The listing builds one solid part. Answer for the finished solid, in the listing's coordinates (mm). Face numbers are marked on the shaded views. Coordinates: 2 decimals unless noted, no trailing zeros. Order: outer loops, then holes, each group sorted by start corner. A loop starts at its lowest first (then second) coordinate and runs counter-clockwise, first axis right, second up.
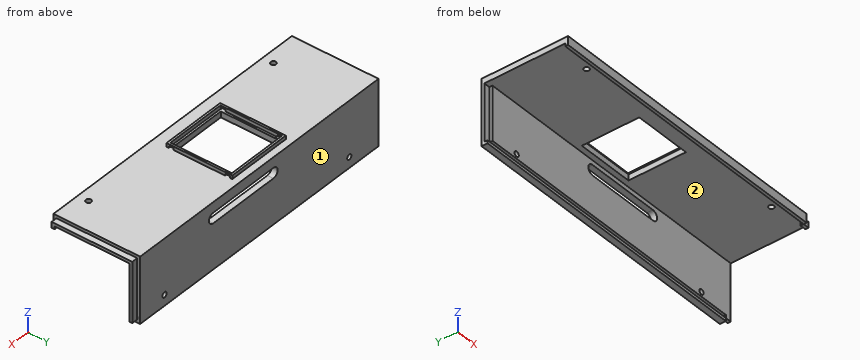
```python
from build123d import *

# Parameters (mm, degrees)
SKETCH_W        = 250
SKETCH_H        = 5
PAD012_DEPTH    = 55
SKETCH023_W     = 2.6
SKETCH023_H     = 2.6
POCKET007_DEPTH = 250.001
SKETCH024_W     = 5.1
SKETCH024_H     = 2.6
POCKET008_DEPTH = 45
SKETCH025_W     = 250
SKETCH025_H     = 4.9
PAD013_DEPTH    = 67.5
SKETCH026_W     = 250
SKETCH026_H     = 2.4
PAD014_DEPTH    = 2.4
SKETCH027_R     = 2.2
HOLE004_DEPTH   = 23.678107
HOLE004_TIPS_R  = 2.2
SKETCH028_R     = 2.2
HOLE005_DEPTH   = 23.678107
HOLE005_TIPS_R  = 2.2
POCKET009_DEPTH = 5
SKETCH030_W     = 48
SKETCH030_H     = 48
POCKET010_DEPTH = 4.9
SKETCH031_W     = 55
SKETCH031_H     = 55
SKETCH031_W_2   = 51.5
SKETCH031_H_2   = 51.5
PAD015_DEPTH    = 3
SKETCH032_W     = 4
SKETCH032_H     = 1.5
POCKET011_DEPTH = 161.951
POCKET012_DEPTH = 5
SKETCH035_W     = 5
SKETCH035_H     = 2.5
PAD016_DEPTH    = 2.6
SKETCH036_W     = 5
SKETCH036_H     = 2.6
PAD017_DEPTH    = 2.4


with BuildPart() as part:
    # Sketch → Pad012 (new body)
    with BuildSketch(Plane.XY):
        with Locations((0, 35)):
            Rectangle(SKETCH_W, SKETCH_H)
    extrude(amount=PAD012_DEPTH)

    # Sketch023 (on Face2 of Pad012) → Pocket007 (cut, through all)
    with BuildSketch(Plane.YZ.offset(125)):
        with Locations((33.8, 3.8)):
            Rectangle(SKETCH023_W, SKETCH023_H)
    extrude(amount=-POCKET007_DEPTH, mode=Mode.SUBTRACT)

    # Sketch024 (on Face7 of Pocket007) → Pocket008 (cut)
    with BuildSketch(Plane(origin=(0, 0, 5.1), x_dir=(1, 0, 0), z_dir=(0, 0, -1))):
        with Locations((-122.45, -33.8)):
            Rectangle(SKETCH024_W, SKETCH024_H)
    extrude(amount=-POCKET008_DEPTH, mode=Mode.SUBTRACT)

    # Sketch025 (on Face6 of Pocket008) → Pad013 (join)
    with BuildSketch(Plane.XZ.offset(-32.5)):
        with Locations((0, 52.55)):
            Rectangle(SKETCH025_W, SKETCH025_H)
    extrude(amount=PAD013_DEPTH)

    # Sketch026 (on Face16 of Pad013) → Pad014 (join)
    with BuildSketch(Plane(origin=(0, 0, 50.1), x_dir=(1, 0, 0), z_dir=(0, 0, -1))):
        with Locations((0, 33.8)):
            Rectangle(SKETCH026_W, SKETCH026_H)
    extrude(amount=PAD014_DEPTH)

    # Sketch027 (on Face1 of Pad014) → Hole004 (cut)
    with BuildSketch(Plane(origin=(0, 37.5, 0), x_dir=(-1, 0, 0), z_dir=(0, 1, 0))):
        with Locations((-95, 9)):
            Circle(SKETCH027_R)
        with Locations((95, 9)):
            Circle(SKETCH027_R)
    extrude(amount=-HOLE004_DEPTH, mode=Mode.SUBTRACT)

    # Hole004 tips → Hole004 tip 1 section 0
    with BuildSketch(Plane(origin=(0, 13.821893, 0), x_dir=(-1, 0, 0), z_dir=(0, 1, 0)), mode=Mode.PRIVATE) as hole004_tip_1_s0:
        with Locations((-95, 9)):
            Circle(HOLE004_TIPS_R)
    loft([hole004_tip_1_s0.sketch, Vertex(95, 12.5, 9)], mode=Mode.SUBTRACT)

    # Hole004 tips → Hole004 tip 2 section 0
    with BuildSketch(Plane(origin=(0, 13.821893, 0), x_dir=(-1, 0, 0), z_dir=(0, 1, 0)), mode=Mode.PRIVATE) as hole004_tip_2_s0:
        with Locations((95, 9)):
            Circle(HOLE004_TIPS_R)
    loft([hole004_tip_2_s0.sketch, Vertex(-95, 12.5, 9)], mode=Mode.SUBTRACT)

    # Sketch028 (on Face14 of Hole004) → Hole005 (cut)
    with BuildSketch(Plane.XY.offset(55)):
        with Locations((-95, -26)):
            Circle(SKETCH028_R)
        with Locations((95, -26)):
            Circle(SKETCH028_R)
    extrude(amount=-HOLE005_DEPTH, mode=Mode.SUBTRACT)

    # Hole005 tips → Hole005 tip 1 section 0
    with BuildSketch(Plane.XY.offset(31.321893), mode=Mode.PRIVATE) as hole005_tip_1_s0:
        with Locations((-95, -26)):
            Circle(HOLE005_TIPS_R)
    loft([hole005_tip_1_s0.sketch, Vertex(-95, -26, 30)], mode=Mode.SUBTRACT)

    # Hole005 tips → Hole005 tip 2 section 0
    with BuildSketch(Plane.XY.offset(31.321893), mode=Mode.PRIVATE) as hole005_tip_2_s0:
        with Locations((95, -26)):
            Circle(HOLE005_TIPS_R)
    loft([hole005_tip_2_s0.sketch, Vertex(95, -26, 30)], mode=Mode.SUBTRACT)

    # Sketch029 (on Face1 of Hole005) → Pocket009 (cut)
    with BuildSketch(Plane(origin=(0, 37.5, 0), x_dir=(-1, 0, 0), z_dir=(0, 1, 0))):
        with BuildLine():
            ThreePointArc((-45, 46.3), (-49.3, 42), (-45, 37.7))
            Line((-45, 37.7), (17, 37.7))
            ThreePointArc((17, 37.7), (21.3, 42), (17, 46.3))
            Line((-45, 46.3), (17, 46.3))
        make_face()
    extrude(amount=-POCKET009_DEPTH, mode=Mode.SUBTRACT)

    # Sketch030 (on Face18 of Pocket009) → Pocket010 (cut)
    with BuildSketch(Plane.XY.offset(55)):
        with Locations((-9.45, 4.09)):
            Rectangle(SKETCH030_W, SKETCH030_H)
    extrude(amount=-POCKET010_DEPTH, mode=Mode.SUBTRACT)

    # Sketch031 (on Face18 of Pocket010) → Pad015 (join)
    with BuildSketch(Plane.XY.offset(55)):
        with Locations((-9.45, 4.09)):
            Rectangle(SKETCH031_W, SKETCH031_H)
        with Locations((-9.45, 4.09)):
            Rectangle(SKETCH031_W_2, SKETCH031_H_2, mode=Mode.SUBTRACT)
    extrude(amount=PAD015_DEPTH)

    # Sketch032 (on Face30 of Pad015) → Pocket011 (cut, through all)
    with BuildSketch(Plane(origin=(-36.95, 0, 0), x_dir=(0, -1, 0), z_dir=(-1, 0, 0))):
        with Locations((-27.59, 55.75)):
            Rectangle(SKETCH032_W, SKETCH032_H)
        with Locations((19.41, 55.75)):
            Rectangle(SKETCH032_W, SKETCH032_H)
    extrude(amount=-POCKET011_DEPTH, mode=Mode.SUBTRACT)

    # Sketch033 (on Face21 of Pocket011) → Pocket012 (cut)
    with BuildSketch(Plane.YZ.offset(125)):
        Polygon((-32.6, 47.7), (-35, 47.7), (-35, 55), (37.5, 55), (37.5, 0), (32.5, 0), (32.5, 2.5), (35, 2.5), (35, 52.55), (-32.6, 52.55), align=None)
    extrude(amount=-POCKET012_DEPTH, mode=Mode.SUBTRACT)

    # Sketch035 (on Face17 of Pocket012) → Pad016 (join)
    with BuildSketch(Plane(origin=(0, 0, 5.1), x_dir=(1, 0, 0), z_dir=(0, 0, -1))):
        with Locations((122.5, -33.75)):
            Rectangle(SKETCH035_W, SKETCH035_H)
    extrude(amount=PAD016_DEPTH)

    # Sketch036 (on Face31 of Pad016) → Pad017 (join)
    with BuildSketch(Plane(origin=(0, 0, 50.1), x_dir=(1, 0, 0), z_dir=(0, 0, -1))):
        with Locations((122.5, 31.3)):
            Rectangle(SKETCH036_W, SKETCH036_H)
    extrude(amount=PAD017_DEPTH)


solid = part.part
```
(1) Find section A-A (z = 42). Write down the section's boundary in (x, y), and give its area (3 significant figures).
(2) Each of these flat-tipped pins is pushed along its axis until it touches: pin 1 Ø0.8 at (x, z) = (-36, 56) entering from -Y; pin 2 Ø1.9 at (x, y) = (17.5, 27.5) entering from -Z; pin 3 Ø1 at (x, y) = (99, -3.5) entering from +Z; pin 4 Ø1.2 at (x, z) = (17, 55.5) entering from +Y. Where does it stop, or does it pass through?
(3) Find section B-B (x = -14.5). Write down the section's boundary in (y, z).
(4) Consider line 1 (Z direction, x = -95, y = 34); line 2 (Y direction, x = 95, z = 51.4); line 3 (X direction, y = 22, z = 51). Determine where each line is inside the solid, lowest interval first.
(5) The mould has two halves that part along Y. Classify the marked faces 1 and 2: released by +Y, released by -Y, zero draft, split by the parting line, or undercut.
(6) Find section D-D (y = 15.5). Write down the section's boundary in (x, z), and give its area (3 significant figures).
(7) Find section C-C (z = 9). Write down the section's boundary in (x, y), and give its area (3 significant figures).
Findings below:
1. outline: (-125, 35.1) - (-119.9, 35.1) - (-119.9, 32.5) - (-21.3, 32.5) - (-21.3, 37.5) - (-125, 37.5) - close; (49.3, 32.5) - (125, 32.5) - (125, 35) - (120, 35) - (120, 37.5) - (49.3, 37.5) - close
1. area: 871 mm2
2. pin 1: stops at y = -23.41
2. pin 2: stops at z = 50.1
2. pin 3: stops at z = 55
2. pin 4: stops at y = 37.5
3. outline: (-35, 47.7) - (-32.6, 47.7) - (-32.6, 50.1) - (-19.91, 50.1) - (-19.91, 55) - (-21.66, 55) - (-21.66, 58) - (-23.41, 58) - (-23.41, 55) - (-35, 55) - close; (28.09, 50.1) - (32.5, 50.1) - (32.5, 46.3) - (37.5, 46.3) - (37.5, 55) - (31.59, 55) - (31.59, 58) - (29.84, 58) - (29.84, 55) - (28.09, 55) - close; (32.5, 0) - (37.5, 0) - (37.5, 37.7) - (32.5, 37.7) - (32.5, 5.1) - (35.1, 5.1) - (35.1, 2.5) - (32.5, 2.5) - close
4. line 1: z = 0 to 2.5, 5.1 to 6.8, 11.2 to 55
4. line 2: y = -35 to -28.2, -23.8 to 37.5
4. line 3: x = -125 to -33.45, 14.55 to 125
5. face 1: released by +Y
5. face 2: undercut
6. outline: (-125, 50.1) - (-33.45, 50.1) - (-33.45, 55) - (-35.2, 55) - (-35.2, 58) - (-36.95, 58) - (-36.95, 55) - (-125, 55) - close; (14.55, 50.1) - (125, 50.1) - (125, 52.55) - (120, 52.55) - (120, 55) - (18.05, 55) - (18.05, 58) - (16.3, 58) - (16.3, 55) - (14.55, 55) - close
6. area: 988 mm2
7. outline: (-125, 35.1) - (-119.9, 35.1) - (-119.9, 32.5) - (-97.2, 32.5) - (-97.2, 37.5) - (-125, 37.5) - close; (-92.8, 32.5) - (92.8, 32.5) - (92.8, 37.5) - (-92.8, 37.5) - close; (97.2, 32.5) - (125, 32.5) - (125, 35) - (120, 35) - (120, 37.5) - (97.2, 37.5) - close
7. area: 1,180 mm2
